```python
from build123d import *

# Parameters (mm, degrees)
SKETCH3_W          = 1.5
SKETCH3_H          = 10
CUT_EXTRUDE1_DEPTH = 2
CIRPATTERN1_COUNT  = 12


with BuildPart() as part:
    # Sketch1 → Revolve1 (revolve)
    with BuildSketch(Plane.XY, mode=Mode.PRIVATE) as revolve1_sk:
        Polygon((3.2, 8.917647059), (6.75, 8.917647059), (8.2, 8.917647059), (8.2, 7.917647059), (6.75, 7.917647059), (6.75, -2.082352941), (8.2, -2.082352941), (8.2, -3.082352941), (6.75, -3.082352941), (3.2, -3.082352941), align=None)
    revolve(revolve1_sk.sketch.rotate(Axis((0, 0, 0), (0, 1, 0)), 90), axis=Axis((0, 0, 0), (0, 1, 0)))  # turned: the seam where the file's is

    # Sketch3 → Cut-Extrude1 (cut)
    with BuildSketch(Plane(origin=(0, 0, -6.75), x_dir=(-1, 0, 0), z_dir=(0, 0, -1))):
        with Locations((0, 2.917647059)):
            Rectangle(SKETCH3_W, SKETCH3_H)
    cut_extrude1 = extrude(amount=-CUT_EXTRUDE1_DEPTH, mode=Mode.SUBTRACT)

    # CirPattern1: Cut-Extrude1 ×12 about axis
    cirpattern1_axis = Axis((0, 0, 0), (0, 1, 0))
    for i in range(1, CIRPATTERN1_COUNT):
        add(cut_extrude1.rotate(cirpattern1_axis, i * 360 / CIRPATTERN1_COUNT), mode=Mode.SUBTRACT)


solid = part.part
```
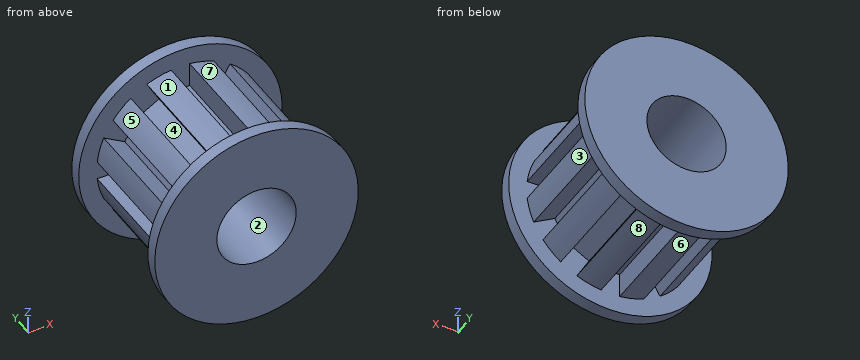
For this review, take the finished solid that the model builds, in its own axes (mm). Face numbers are marked on the shaded views. A direction names the side the tool comes from. Round coordinates to 2 decimals unless told otherwise and drop trailing zeros. Write each loop counter-clockwise with the first axis right and the second up, starting at its lowest first coordinate (ties: lowest second). Pieces come first, ordered by that corner, then holes. Notation, with made-up numbers: (26.25, 15.25) - (79.25, 15.25) arc R24 cw to (79.25, 47.25) - close; hole circle Ø8 at (-30.75, 82). An arc over 180 degrees is marked (long way). Answer as a JSON object with one key per item and string values.
1. For pin 1 Ø5 at (x, y) = (0.5, 6.5) entering from -Z; pin 2 Ø5 at (y, z) = (2.5, -0.5) entering from +X; pin 3 Ø2 at (x, y) = (6.5, 3) entering from +Z; pin 4 Ø1.6 at (x, y) = (-6, 4.5) entering from -Z, all flat-tipped, find the tip position at first contact; note any pin that passes through.
Response values:
{"pin 1": "stops at z = -8.2", "pin 2": "stops at x = 6.71", "pin 3": "stops at z = 2.7", "pin 4": "stops at z = -4.3"}
2. We need section C-C on x = -2.25. Give the boundary of the cut face in (y, z), then the cut area to 3 significant figures.
Response values:
{"outline": "(-3.08, -7.89) - (-2.08, -7.89) - (-2.08, -6.36) - (7.92, -6.36) - (7.92, -7.89) - (8.92, -7.89) - (8.92, -2.28) - (-3.08, -2.28) - close; (-3.08, 2.28) - (8.92, 2.28) - (8.92, 7.89) - (7.92, 7.89) - (7.92, 6.36) - (-2.08, 6.36) - (-2.08, 7.89) - (-3.08, 7.89) - close; hole (-2.08, -5.4) - (7.92, -5.4) - (7.92, -4.19) - (-2.08, -4.19) - close; hole (-2.08, 4.19) - (7.92, 4.19) - (7.92, 5.4) - (-2.08, 5.4) - close", "area": "80.0 mm2"}
3. We need section A-A on x = 0. Give the boundary of the cut face in (y, z).
Response values:
{"outline": "(-3.08, -8.2) - (-2.08, -8.2) - (-2.08, -4.75) - (7.92, -4.75) - (7.92, -8.2) - (8.92, -8.2) - (8.92, -3.2) - (-3.08, -3.2) - close; (-3.08, 3.2) - (8.92, 3.2) - (8.92, 8.2) - (7.92, 8.2) - (7.92, 4.75) - (-2.08, 4.75) - (-2.08, 8.2) - (-3.08, 8.2) - close"}
4. To check wall thickness, follow line 1 along X through (y, z) = (3.25, 0); line 2 along Z through (x, y) = (-4.25, 5); line 3 along X through (y, z) = (7, 5.25). State the ranges of each line that lie inside material, in increasing order.
Response values:
{"line 1": "x = -4.75 to -3.2, 3.2 to 4.75", "line 2": "z = -5.24 to -3.32, -2.14 to 2.14, 3.32 to 5.24", "line 3": "x = -4.24 to -3.9, -2.17 to -0.75, 0.75 to 2.17, 3.9 to 4.24"}
5. We need section D-D on z = 4.25. Give the boundary of the cut face in (x, y), then the cut area to 3 significant figures.
Response values:
{"outline": "(-7.01, -3.08) - (7.01, -3.08) - (7.01, -2.08) - (5.24, -2.08) - (5.24, 7.92) - (7.01, 7.92) - (7.01, 8.92) - (-7.01, 8.92) - (-7.01, 7.92) - (-5.24, 7.92) - (-5.24, -2.08) - (-7.01, -2.08) - close; hole (-3.32, -2.08) - (-2.14, -2.08) - (-2.14, 7.92) - (-3.32, 7.92) - close; hole (2.14, -2.08) - (3.32, -2.08) - (3.32, 7.92) - (2.14, 7.92) - close", "area": "109 mm2"}
6. Tool access review of the marked faces 5, 6, 7 and 8: name each direction out of +Z, -Z, +X, -X, +Y, -Y from which nothing blocks a thin tool from reaching the whole face with its end or side.
Response values:
{"face 5": "+Z, -X", "face 6": "-Z, -X", "face 7": "+Z, +X", "face 8": "-Z, +X"}
7. We need section B-B on z = 0. Give the boundary of the cut face in (x, y), then the cut area to 3 significant figures.
Response values:
{"outline": "(-8.2, -3.08) - (-3.2, -3.08) - (-3.2, 8.92) - (-8.2, 8.92) - (-8.2, 7.92) - (-4.75, 7.92) - (-4.75, -2.08) - (-8.2, -2.08) - close; (3.2, -3.08) - (8.2, -3.08) - (8.2, -2.08) - (4.75, -2.08) - (4.75, 7.92) - (8.2, 7.92) - (8.2, 8.92) - (3.2, 8.92) - close", "area": "51.0 mm2"}
8. Draft analysis for pull direction X (two halves, no side actions). For the marked faces 1, 2, 3 and 4, state which applies: +X half, -X half, draft (parallel to the pull), parting line (faces both ways), or undercut.
Response values:
{"face 1": "-X half", "face 2": "undercut", "face 3": "+X half", "face 4": "undercut"}
